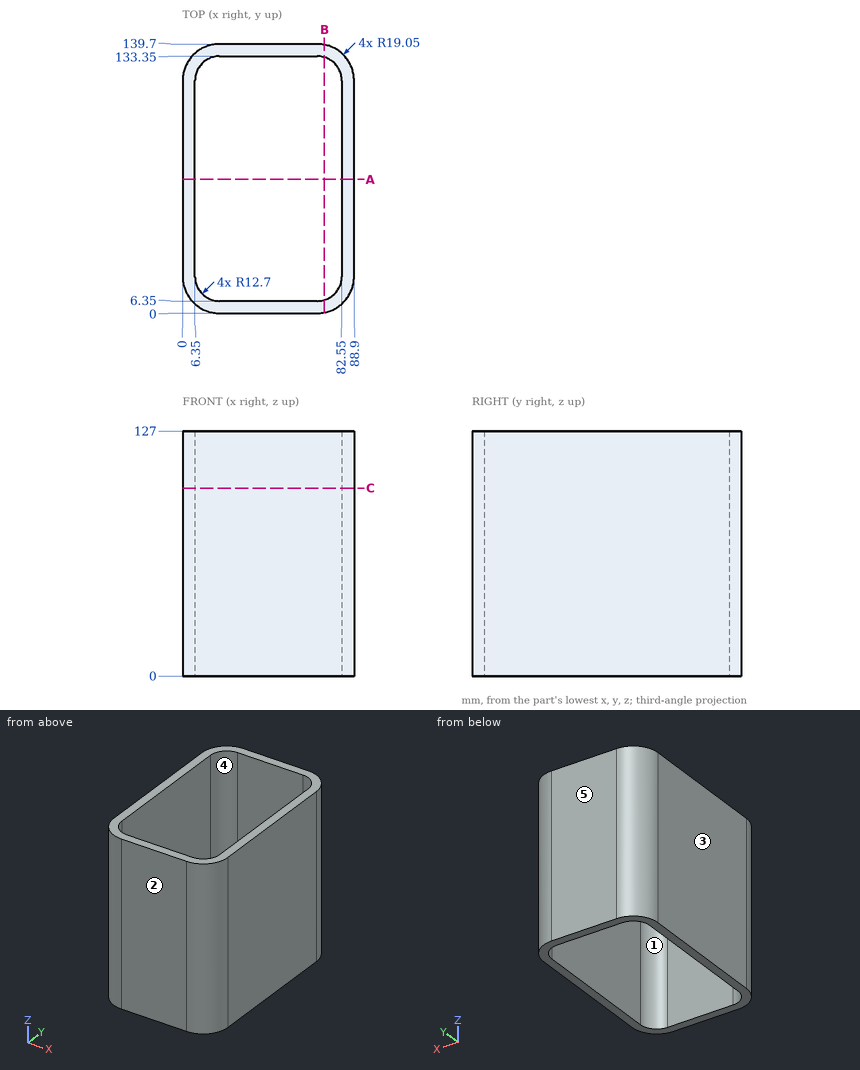
Design review of the part shown in the three views and the two pictorial views. Dimensions are in mm from the part's minimum x, y and z. A direction names the side the tool comes from. Coordinates: 2 decimals unless noted, no trailing zeros. Write each loop counter-clockwise with the first axis right and the second up, starting at its lowest first coordinate (ties: lowest second). Pieces come first, ordered by that corner, then holes. Notation, with made-up numbers: (-28.5, -33) - (19.5, -33) arc R31 ccw to (19.5, -2) - close; hole circle Ø10 at (62, 82). An arc over 180 degrees is marked (long way). Write item = value, one per line.
(1) For P1, Ø6, axis at x = 10.5, z = 27, coming from the +Y side; P2, Ø4, axis at x = 78.5, z = 27.5, coming from the -Y side; P3, Ø5, axis at y = 14.5, z = 89.5, coming from the -X side, all flat-tipped, find the tip position at first contact; note any pin that passes through.
Result sheet:
P1 = 138.87
P2 = 1.2
P3 = 0.11
(2) Consider section A-A, the plane y = 69.5. Give the boundary of the cut face in (x, z), then the cut area to 3 significant figures.
Result sheet:
outline = (0, 0) - (6.35, 0) - (6.35, 127) - (0, 127) - close; (82.55, 0) - (88.9, 0) - (88.9, 127) - (82.55, 127) - close
area = 1,610 mm^2
(3) For line 1 (X direction, y = 52.5, z = 57); line 2 (Y direction, x = 34, z = 29); line 3 (Y direction, x = 77, z = 50.5), list the stretches that pass through material, from the lowest coordinate up. Write a range as [from, to].
Result sheet:
line_1 = [0, 6.35], [82.55, 88.9]
line_2 = [0, 6.35], [133.35, 139.7]
line_3 = [1.39, 8.55], [131.15, 138.31]
(4) Consider section B-B, the plane x = 73.5. Give the boundary of the cut face in (y, z).
Result sheet:
outline = (0.35, 0) - (6.89, 0) - (6.89, 127) - (0.35, 127) - close; (132.81, 0) - (139.35, 0) - (139.35, 127) - (132.81, 127) - close
(5) Machinability: for the marked faces 1 and 2, which of the approach directions +Z, -Z, +X, -X, +Y, -Y give a long, thin tool a straight path to every point of the face, cutting with its end or side? Answer none if there is none.
Result sheet:
face_1 = +Z, -Z
face_2 = +Z, -Z, +X, -X, -Y
(6) Mouldability with a two-part tool opening along X and no side actions: class the marked faces 3, 4 and 5 as pulls with the +X half, pulls with the -X half, needs draft (parallel to the pull), parting line crosses it, or undercut.
Result sheet:
face_3 = pulls with the -X half
face_4 = undercut
face_5 = needs draft
(7) Consider section C-C, the plane z = 97.5. Give the boundary of the cut face in (x, y), then the cut area to 3 significant figures.
Result sheet:
outline = (0, 19.05) arc R19.05 ccw to (19.05, 0) - (69.85, 0) arc R19.05 ccw to (88.9, 19.05) - (88.9, 120.65) arc R19.05 ccw to (69.85, 139.7) - (19.05, 139.7) arc R19.05 ccw to (0, 120.65) - close; hole (6.35, 19.05) arc R12.7 ccw to (19.05, 6.35) - (69.85, 6.35) arc R12.7 ccw to (82.55, 19.05) - (82.55, 120.65) arc R12.7 ccw to (69.85, 133.35) - (19.05, 133.35) arc R12.7 ccw to (6.35, 120.65) - close
area = 2,570 mm^2
